Part model, mm, in its own coordinate system. A direction names the side the tool comes from. Round coordinates to 2 decimals unless told otherwise and drop trailing zeros. Write each loop counter-clockwise with the first axis right and the second up, starting at its lowest first coordinate (ties: lowest second). Pieces come first, ordered by that corner, then holes. Notation, with made-up numbers: M -28.5,27 L 9.5,27 A27 cw 9.5,57 Z; hole C 59,-1.5 d10. An arc over 180 degrees is marked long. Use one line per item in the form item = value. Start each with the question number.
Item 1: Mould opens along X. For faces 1 (the face through (26.5, -12, 15)), 2 (the face through (0, 9.5, 49)), 3 (the face through (-14.68, 11.26, 16.76)), 4 (the face through (14, 0, 17)) say: +X half, -X half, draft (parallel to the pull), parting line (faces both ways), or undercut.
Item 2: Probe L1, parallel to Z at x = -3, y = 1; L2, parallel to Y at x = 8.5, z = 17; L3, parallel to Y at x = -7, z = 18. List the from-to ranges inside material, lowest first.
Item 3: Flat gauge pins, fed straight in: pin 1 Ø9 at (x, z) = (9.5, 20) entering from -Y; pin 2 Ø3.5 at (x, y) = (-15.5, 0) entering from -Z; pin 3 Ø6 at (x, y) = (15, 1) entering from +Z. Where does each tip first touch, or does it go through?
Item 4: Which spindle directions (+Z, -Z, +X, -X, +Y, -Y) get a long thin tool onto all of the face, cutting with end or side? Do faces 5 (the face through (22, 7, 14)), 6 (the face through (-1.15, 4.23, -5.72)), 7 (the face through (9, -18.5, 17)), 8 (the face through (0, 7, 55)), 9 (the face through (-6, 7, 37)). Say none if no direction does.
Item 5: Cut at A-A, the plane y = 0. Give the cut face in (x, z).
Item 6: Cut at C-C, the plane z = 27. Give the cut face in (x, y).
Item 7: Cut at D-D, the plane y = -6.5. Give the cut face in (x, z), then the cut area to 3 significant figures.
Item 8: Cut at B-B, the plane x = -7.75. Give the cut face in (y, z), then the cut area to 3 significant figures.
Solid Edge part; units mm, degrees
sketch "Sketch1" plane through (0, 0, 0) normal (0, 0, 1) x (1, 0, 0)
  circle A0 centre (0, 0) radius 18.5
extrude "Protrusion1" add sketch "Sketch1" along normal blind 34
sketch "Sketch2" plane through (0, 0, 34) normal (0, 0, 1) x (1, 0, 0)
  circle A0 centre (0, 7) radius 6
extrude "ExtrudedProtrusion_2" add sketch "Sketch2" along normal blind 6
sketch "Sketch3" plane through (0, 7, 40) normal (0, 0, 1) x (1, 0, 0)
  circle A0 centre (0, 0) radius 3
extrude "ExtrudedProtrusion_3" add sketch "Sketch3" along normal blind 15
sketch "Sketch4" plane through (0, 7, 55) normal (0, 0, 1) x (1, 0, 0)
  line L0 (-1.6583, 2.5) -> (1.6583, 2.5)
extrude "ExtrudedCutout_1" cut sketch "Sketch4" against normal blind 13 material side at (0, 9.55, 55)
sketch "Sketch5" plane through (0, 0, 0) normal (0, 0, -1) x (0, -1, 0)
  circle A0 centre (-7, 0) radius 3
extrude "ExtrudedProtrusion_4" add sketch "Sketch5" along normal blind 11.6
sketch "Sketch6" plane through (0, 0, 0) normal (1, 0, 0) x (0, 1, 0)
  line L0 (-18.5, 0) -> (7, 0)
  line L1 (7, 0) -> (7, 33.5)
  line L2 (7, 33.5) -> (-18.5, 33.5)
  line L3 (-18.5, 33.5) -> (-18.5, 0)
  dimension "D1" = 18.5
extrude "ExtrudedProtrusion_5" add sketch "Sketch6" along normal blind 18.5
sketch "Sketch7" plane through (18.5, -5.75, 16.75) normal (1, 0, 0) x (0, 0, -1)
  line L0 (-16.75, 12.75) -> (21.75, 12.75)
  line L1 (21.75, 12.75) -> (21.75, -23.85)
  line L2 (21.75, -23.85) -> (-16.75, -23.85)
  line L3 (-16.75, -23.85) -> (-16.75, 12.75)
extrude "ExtrudedProtrusion_6" add sketch "Sketch7" along normal blind 8
hole "Hole_1" at (-7.75, 13.4234, 34) direction (0, 0, -1) diameter 3 end through all
pattern_circular "Pattern1" count 6 over 360 about axis through (0, 0, 34) along (0, 0, -1) of "Hole_1"
hole "Hole_7" at (26.5, -11.3, 14.25) direction (-1, 0, 0) diameter 0.1 depth 140
Model answer:
q1.face_1 = +X half
q1.face_2 = draft
q1.face_3 = parting line
q1.face_4 = undercut
q2.L1 = 0 to 34
q2.L2 = -18.5 to -14.72, -12.12 to 12.12, 14.72 to 16.43
q2.L3 = -17.12 to -14.72, -12.12 to 12.12, 14.72 to 17.12
q3.pin_1 = -18.5
q3.pin_2 = 0
q3.pin_3 = 34
q4.face_5 = +Z, -Z, +X, +Y
q4.face_6 = -Z
q4.face_7 = +Z, -Z, -X, -Y
q4.face_8 = +Z, +X, -X, +Y, -Y
q4.face_9 = +Z
q5.outline = M -18.5,0 L -17,0 L -17,34 L -18.5,34 Z; M -14,0 L 14,0 L 14,34 L -14,34 Z; M 17,0 L 18.5,0 L 18.5,-5 L 26.5,-5 L 26.5,33.5 L 18.5,33.5 L 18.5,34 L 17,34 Z
q6.outline = M 0,-18.5 L 18.5,-18.5 L 18.5,-29.6 L 26.5,-29.6 L 26.5,7 L 17.12,7 A18.5 ccw long Z; hole C -15.5,0 d3; hole C -7.75,-13.42 d3; hole C -7.75,13.42 d3; hole C 7.75,-13.42 d3; hole C 7.75,13.42 d3; hole C 15.5,0 d3
q7.outline = M -17.32,0 L 18.5,0 L 18.5,-5 L 26.5,-5 L 26.5,33.5 L 17.32,33.5 L 17.32,34 L -17.32,34 Z
q7.area = 1,530 mm²
q8.outline = M -16.8,0 L -14.92,0 L -14.92,34 L -16.8,34 Z; M -11.92,0 L 11.92,0 L 11.92,34 L -11.92,34 Z; M 14.92,0 L 16.8,0 L 16.8,34 L 14.92,34 Z; hole C -11.3,14.25 d0.1
q8.area = 938 mm²
